Design review of the part built by this model. Coordinates are the model's own, in mm. Face numbers are marked on the shaded views. A direction names the side the tool comes from. Coordinates: 2 decimals unless noted, no trailing zeros. Write each loop counter-clockwise with the first axis right and the second up, starting at its lowest first coordinate (ties: lowest second). Pieces come first, ordered by that corner, then holes.
Q1. Take a section at A-A (z = -23). Give the boundary of the cut face in (x, y).
Q2. Machinability: for the marked faces 1, 2 and 3, which of the approach directions +Z, -Z, +X, -X, +Y, -Y give a long, thin tool a straight path to every point of the face, cutting with its end or side? Answer none if there is none.
Q3. For probe 1 along X at (y, z) = (1, -56.5); probe 2 along X at (y, z) = (-6, 24.7); probe 3 along X at (y, z) = (-6.45, 36.2), list the stretches that pass through material, from the lowest coordinate up.
Q4. Take a section at D-D (x = 34.5). Give the boundary of the cut face in (y, z).
Q5. Take a section at B-B (x = 7). Give the boundary of the cut face in (y, z).
Q6. Insertion check: pin 1 (4.5 mm diameter, centred on x = 3.5, z = 60.5, fed in from +Y); pin 2 (0.9 mm diameter, centred on x = 44.5, y = -1.5, fed in from +Z); pin 3 (2.5 mm diameter, centred on x = 16.5, y = -3.5, fed in from -Z); pin 4 (6 mm diameter, centred on x = 3.5, z = -56.5, fed in from +Y). Each pin has a flat end and moves straight along its axis. Give the tip position at first contact, or say it passes through.
Q7. Take a section at C-C (z = 60.5). Give the boundary of the cut face in (x, y).
```python
from build123d import *

# Parameters (mm, degrees)
BOSS_EXTRUDE1_DEPTH = 61.34
SKETCH3_R           = 13
SKETCH3_R_2         = 1.9
CUT_EXTRUDE1_DEPTH  = 90.104408421
SKETCH4_R           = 6.5
SKETCH4_R_2         = 1.9
CUT_EXTRUDE2_DEPTH  = 89.924662496
FILLET1_R           = 2
FILLET3_R           = 2


with BuildPart() as part:
    # Sketch2 → Boss-Extrude1 (new body)
    with BuildSketch(Plane(origin=(0, 0, 0), x_dir=(0, 0, -1), z_dir=(1, 0, 0))):
        Polygon((0, 0), (60, 0), (60, 2), (-2, 2), (-2, -5), (-64, -5), (-64, -7), (0, -7), align=None)
    extrude(amount=BOSS_EXTRUDE1_DEPTH)

    # Sketch3 → Cut-Extrude1 (cut, through all)
    with BuildSketch(Plane(origin=(0, 2, 0), x_dir=(1, 0, 0), z_dir=(0, 1, 0))):
        with Locations(Location((27.5, 23, 0), (0, 0, 270))):
            Circle(SKETCH3_R)
        with Locations(Location((57.84, 56.5, 0), (0, 0, 270))):
            Circle(SKETCH3_R_2)
        with Locations(Location((3.5, 56.5, 0), (0, 0, 270))):
            Circle(SKETCH3_R_2)
    extrude(amount=-CUT_EXTRUDE1_DEPTH, mode=Mode.SUBTRACT)

    # Sketch4 → Cut-Extrude2 (cut, through all)
    with BuildSketch(Plane(origin=(0, -5, 0), x_dir=(1, 0, 0), z_dir=(0, 1, 0))):
        with Locations(Location((38.07, -24.7, 0), (0, 0, 270))):
            Circle(SKETCH4_R)
        with Locations(Location((26.57, -36.2, 0), (0, 0, 270))):
            Circle(SKETCH4_R)
        with Locations(Location((15.07, -24.7, 0), (0, 0, 270))):
            Circle(SKETCH4_R)
        with Locations(Location((26.57, -13.2, 0), (0, 0, 270))):
            Circle(SKETCH4_R)
        with Locations(Location((57.84, -60.5, 0), (0, 0, 270))):
            Circle(SKETCH4_R_2)
        with Locations(Location((3.5, -60.5, 0), (0, 0, 270))):
            Circle(SKETCH4_R_2)
    extrude(amount=-CUT_EXTRUDE2_DEPTH, mode=Mode.SUBTRACT)

    # Fillet1
    fillet1_edges = [part.edges().sort_by_distance(p)[0] for p in [
        (30.67, -7, 0),
        (30.67, -5, 2),
        (30.67, 2, 2),
        (30.67, 0, 0),
    ]]
    fillet(fillet1_edges, radius=FILLET1_R)

    # Fillet3
    fillet3_edges = [part.edges().sort_by_distance(p)[0] for p in [
        (0, 1, -60),
        (61.34, 1, -60),
        (61.34, -6, 64),
        (0, -6, 64),
    ]]
    fillet(fillet3_edges, radius=FILLET3_R)


solid = part.part
```
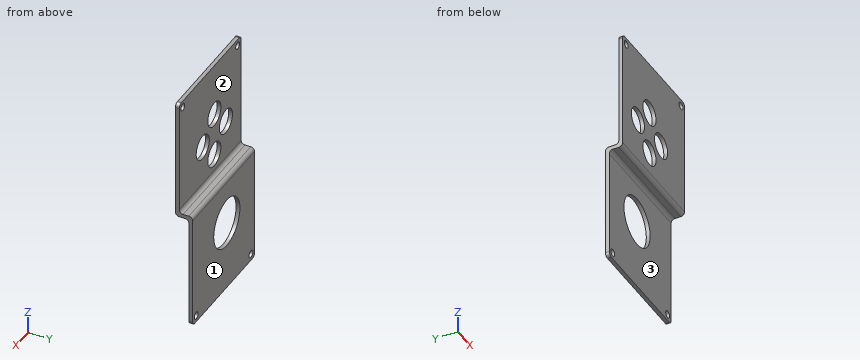
Response:
1. outline: (0, 0) - (14.5, 0) - (14.5, 2) - (0, 2) - close; (40.5, 0) - (61.34, 0) - (61.34, 2) - (40.5, 2) - close
2. face 1: +Z, -Z, +X, -X, +Y
2. face 2: +Z, +X, -X, +Y
2. face 3: -Z, +X, -X, -Y
3. probe 1: x = 0 to 1.6, 5.4 to 55.94, 59.74 to 61.34
3. probe 2: x = 0 to 8.57, 21.57 to 31.57, 44.57 to 61.34
3. probe 3: x = 0 to 20.07, 33.07 to 61.34
4. outline: (-7, 2) arc R2 ccw to (-5, 0) - (-2, 0) arc R2 cw to (0, -2) - (0, -12.05) - (2, -12.05) - (2, 0) arc R2 ccw to (0, 2) - (-3, 2) arc R2 cw to (-5, 4) - (-5, 19.27) - (-7, 19.27) - close; (-7, 30.13) - (-5, 30.13) - (-5, 64) - (-7, 64) - close; (0, -60) - (2, -60) - (2, -33.95) - (0, -33.95) - close
5. outline: (-7, 2) arc R2 ccw to (-5, 0) - (-2, 0) arc R2 cw to (0, -2) - (0, -60) - (2, -60) - (2, 0) arc R2 ccw to (0, 2) - (-3, 2) arc R2 cw to (-5, 4) - (-5, 64) - (-7, 64) - close
6. pin 1: stops at y = -5
6. pin 2: stops at z = 2
6. pin 3: stops at z = 0
6. pin 4: stops at y = 2
7. outline: (0, -7) - (1.6, -7) - (1.6, -5) - (0, -5) - close; (5.4, -7) - (55.94, -7) - (55.94, -5) - (5.4, -5) - close; (59.74, -7) - (61.34, -7) - (61.34, -5) - (59.74, -5) - close
